Verification items for this drawing (mm, ordinates from the low corner). Give positions to 0.01 mm unless a question says otherwise; leave off trailing zeros. Loops run counter-clockwise (first coordinate to the right, second up) from the corner with the lowest first, then second, coordinate; pieces in that order, holes last. Notation, with made-up numbers: (-1.75, 4) -> (51.25, 4) arc R25 ccw to (51.25, 30) -> close; hole circle Ø4 at (-38.5, 58). An arc over 180 degrees is marked (long way). Use one line per item in the form item = value. Start each with the question number.
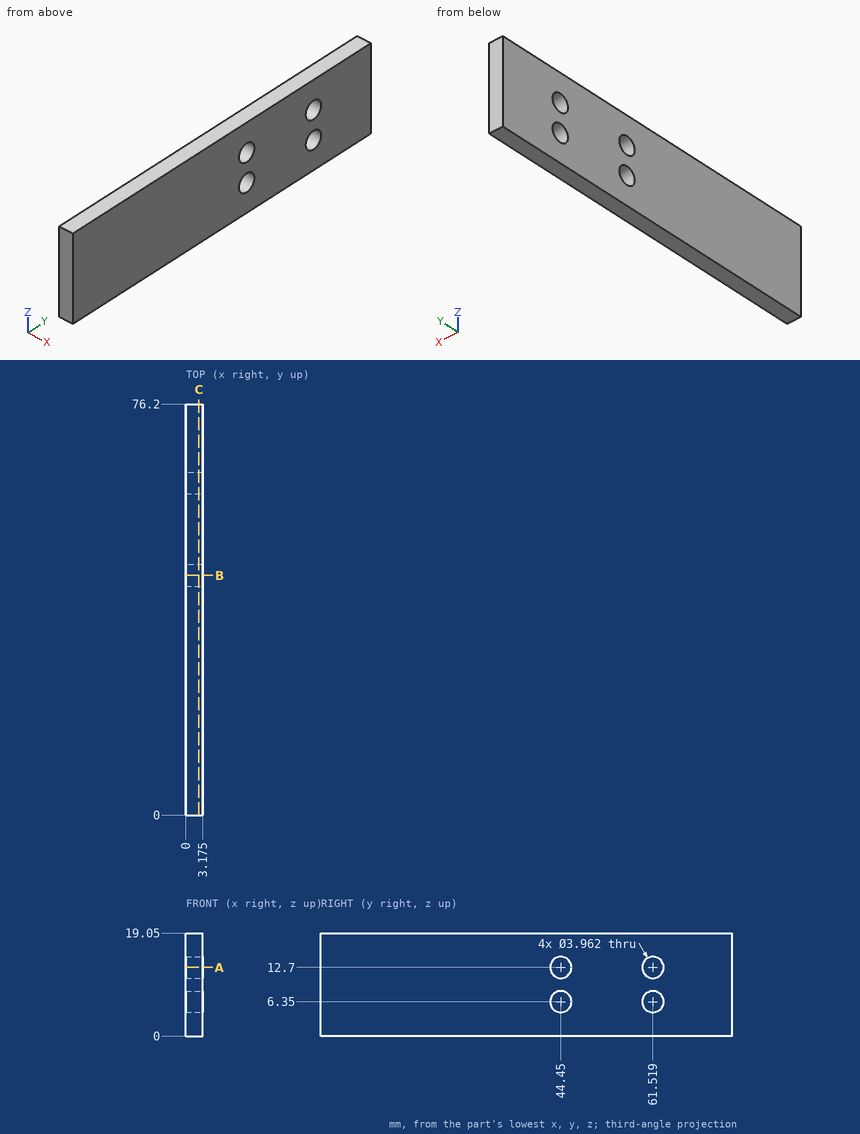
Item 1: Sectioned sample at B-B, the plane y = 44.45. State how many separate pieces and enclosed holes the cut face has.
Item 2: Sectioned sample at A-A, the plane z = 12.7. Enter the section's corners in (x, y) (1 decimal).
Item 3: Sectioned sample at C-C, the plane x = 2.4. Enter the section's corners in (y, z), and give its area (3 significant figures).
Item 4: Material ranges on line 1 (Z direction, x = 2.35, y = 44.45); line 2 (Y direction, x = 2.3, z = 12.5); line 3 (Y direction, x = 0.6, z = 5), recorded low to high.
Outcome:
q1.separate_pieces = 3
q1.enclosed_holes = 0
q2.outline = (0, 0) -> (3.2, 0) -> (3.2, 42.5) -> (0, 42.5) -> close; (0, 46.4) -> (3.2, 46.4) -> (3.2, 59.5) -> (0, 59.5) -> close; (0, 63.5) -> (3.2, 63.5) -> (3.2, 76.2) -> (0, 76.2) -> close
q3.outline = (0, 0) -> (76.2, 0) -> (76.2, 19.05) -> (0, 19.05) -> close; hole circle Ø3.96 at (44.45, 6.35); hole circle Ø3.96 at (44.45, 12.7); hole circle Ø3.96 at (61.52, 6.35); hole circle Ø3.96 at (61.52, 12.7)
q3.area = 1,400 mm^2
q4.line_1 = 0 to 4.37, 8.33 to 10.72, 14.68 to 19.05
q4.line_2 = 0 to 42.48, 46.42 to 59.55, 63.49 to 76.2
q4.line_3 = 0 to 43, 45.9 to 60.07, 62.97 to 76.2
